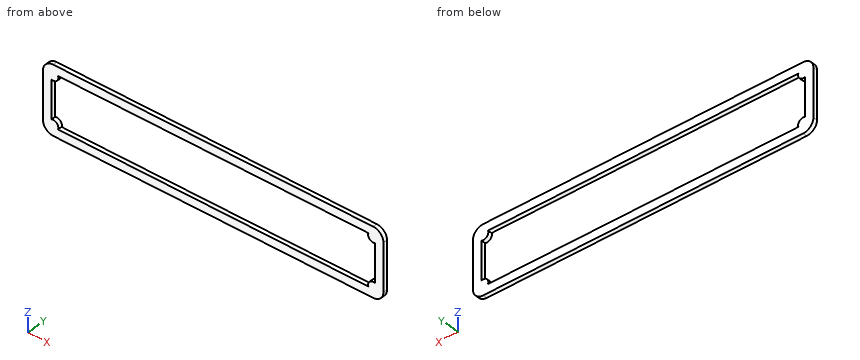
```python
from build123d import *

# Parameters (mm, degrees)
F0_W     = 254
F0_H     = 50.8
F1_DEPTH = 3.175
F2_R     = 7.62
F4_DEPTH = 25.4
F5_R     = 3.81
F6_DEPTH = 3.175


with BuildPart() as f1:
    # F0 (on Front) → F1 (new body)
    with BuildSketch(Plane.XZ):
        Rectangle(F0_W, F0_H)
    extrude(amount=F1_DEPTH)

    # F2
    f2_edges = [f1.edges().sort_by_distance(p)[0] for p in [
        (-127, -1.5875, 25.4),
        (-127, -1.5875, -25.4),
        (127, -1.5875, 25.4),
        (127, -1.5875, -25.4),
    ]]
    fillet(f2_edges, radius=F2_R)

    # F3 (on face) → F4 (cut)
    with BuildSketch(Plane.XZ.offset(3.175)):
        with BuildLine():
            Line((119.38, 19.05), (-119.38, 19.05))
            ThreePointArc((-119.38, 19.05), (-120.278026, 18.678026), (-120.65, 17.78))
            Line((-120.65, 17.78), (-120.65, -17.78))
            ThreePointArc((-120.65, -17.78), (-120.278026, -18.678026), (-119.38, -19.05))
            Line((-119.38, -19.05), (119.38, -19.05))
            ThreePointArc((119.38, -19.05), (120.278026, -18.678026), (120.65, -17.78))
            Line((120.65, -17.78), (120.65, 17.78))
            ThreePointArc((120.65, 17.78), (120.278026, 18.678026), (119.38, 19.05))
        make_face()
    extrude(amount=-F4_DEPTH, mode=Mode.SUBTRACT)

    # F5 (on face) → F6 (join)
    with BuildSketch(Plane.XZ.offset(3.175)):
        with Locations((-119.38, 17.78)):
            Circle(F5_R)
        with Locations((-119.38, -17.78)):
            Circle(F5_R)
        with Locations((119.38, 17.78)):
            Circle(F5_R)
        with Locations((119.38, -17.78)):
            Circle(F5_R)
    extrude(amount=-F6_DEPTH)


solid = f1.part
```
Check sheet for the modelled part. Datum: model origin and axes. Units: mm. Round coordinates to 2 decimals unless told otherwise and drop trailing zeros. Order: outer loops, then holes, each group sorted by start corner. A loop starts at its lowest first (then second) coordinate and runs counter-clockwise, first axis right, second up. Notation, with made-up numbers: M -37.75,79.25 L 7.25,79.25 A21 ccw 7.25,118.25 Z; hole C -25,21 d9. An arc over 180 degrees is marked long. Answer in a Markdown table with one row per item.
(1) Section check B-B on x = 72.5. Record the boundary of the cut face in (y, z) (3 decimals), plus the area to 3 significant figures.
Findings:
| item | result |
|---|---|
| outline | M -3.175,-25.4 L 0,-25.4 L 0,-19.05 L -3.175,-19.05 Z; M -3.175,19.05 L 0,19.05 L 0,25.4 L -3.175,25.4 Z |
| area | 40.3 mm^2 |
(2) Section check C-C on z = -2. Record the boundary of the cut face in (x, y) (3 decimals).
Findings:
| item | result |
|---|---|
| outline | M -127,-3.175 L -120.65,-3.175 L -120.65,0 L -127,0 Z; M 120.65,-3.175 L 127,-3.175 L 127,0 L 120.65,0 Z |
(3) Material ranges on line 1 along Z through (x, y) = (40, -2.4); line 2 along X through (y, z) = (-1.85, 18); line 3 along X through (y, z) = (-1.5, 10), recorded low to high. Write a range as from..to.
Findings:
| item | result |
|---|---|
| line 1 | z = -25.4..-19.05, 19.05..25.4 |
| line 2 | x = -127..-115.58, 115.58..127 |
| line 3 | x = -127..-120.65, 120.65..127 |
(4) Section check A-A on y = -0.8. Record the boundary of the cut face in (x, z), plus the area to 3 significant figures.
Findings:
| item | result |
|---|---|
| outline | M -127,-17.78 A7.62 ccw -119.38,-25.4 L 119.38,-25.4 A7.62 ccw 127,-17.78 L 127,17.78 A7.62 ccw 119.38,25.4 L -119.38,25.4 A7.62 ccw -127,17.78 Z; hole M -120.65,-14.19 A3.81 cw -115.79,-19.05 L 115.79,-19.05 A3.81 cw 120.65,-14.19 L 120.65,14.19 A3.81 cw 115.79,19.05 L -115.79,19.05 A3.81 cw -120.65,14.19 Z |
| area | 3,750 mm^2 |
